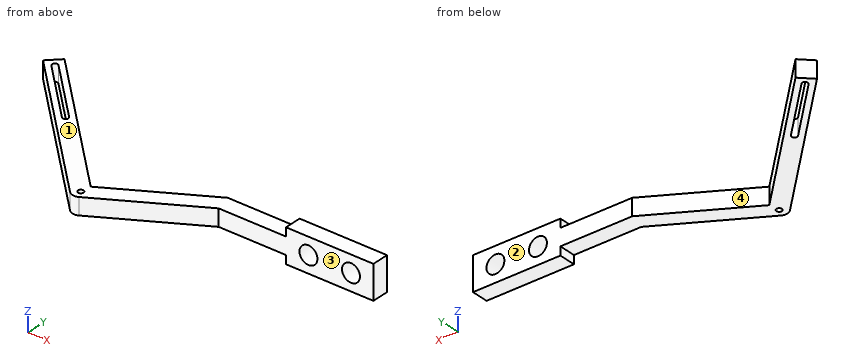
Autodesk Inventor part; units mm, degrees
ref_plane "YZ Plane" through (0, 0, 0) normal (1, 0, 0) x (0, 1, 0)
ref_plane "XZ Plane" through (0, 0, 0) normal (0, 1, 0) x (-1, 0, 0)
ref_plane "XY Plane" through (0, 0, 0) normal (0, 0, 1) x (1, 0, 0)
sketch "Sketch1" plane through (0, 0, 0) normal (0, 0, 1) x (1, 0, 0)
  line L0 (37.3205, 11.5) -> (16.9186, 11.5)
  line L1 (-26.163, 24.0416) -> (-1.0607, -1.0607)
  line L2 (17.7224, 8.5) -> (0.75, -1.299)
  line L3 (17.7224, 8.5) -> (37.3205, 8.5)
  line L4 (0.2468, 1.8745) -> (16.9186, 11.5)
  line L5 (0.2468, 1.8745) -> (-24.0416, 26.163)
  arc A0 (-23.6881, 24.3952) -> (-24.3952, 23.6881) centre (-24.0416, 24.0416) ccw
  arc A1 (-14.4957, 13.7886) -> (-13.7886, 14.4957) centre (-14.1421, 14.1421) ccw
  circle A2 centre (0, 0) radius 0.5
  line L6 (-25.1023, 25.1023) -> (-26.163, 24.0416)
  line L7 (-24.0416, 26.163) -> (-25.1023, 25.1023)
  line L8 (-24.3952, 23.6881) -> (-14.4957, 13.7886)
  line L9 (-13.7886, 14.4957) -> (-23.6881, 24.3952)
  line L10 (37.3205, 8.5) -> (45.3205, 8.5)
  line L11 (45.3205, 8.5) -> (45.3205, 11.5)
  line L12 (45.3205, 11.5) -> (37.3205, 11.5)
  arc A3 (-1.0607, -1.0607) -> (0.75, -1.299) centre (0, 0) ccw
extrude "Extrusion1" add sketch "Sketch1" along normal blind 3
sketch "Sketch5" plane through (0, 0, 3) normal (0, 0, 1) x (1, 0, 0)
  point P0 (0, 0)
sketch "Sketch8" plane through (45.3205, 8.5, 0) normal (1, 0, 0) x (0, 0, -1)
  line L0 (0, 0) -> (-3, 0)
  line L1 (-3, 0) -> (-4.5, 0)
  line L2 (-4.5, 0) -> (-4.5, 3)
  line L3 (-4.5, 3) -> (1.5, 3)
  line L4 (1.5, 3) -> (1.5, 0)
  line L5 (1.5, 0) -> (-3, 0)
  point P0 (0, -8.5)
  dimension "d38" = 1.5
  dimension "d39" = 3
  dimension "d40" = 6
  dimension "d41" = 3
extrude "Extrusion4" add sketch "Sketch8" against normal blind 15.588
sketch "Sketch9" plane through (16.9186, 11.5, 3) normal (0, 1, 0) x (1, 0, 0)
  line L0 (28.4019, 4.5) -> (28.4019, -1.5) construction
  point P0 (-16.9186, 3)
  point P1 (24.4019, 1.5)
  point P2 (16.8139, 1.5)
hole "Hole2" at (41.3205, 11.5, 1.5) at (33.7325, 11.5, 1.5) direction (0, -1, 0) diameter 3.2 end through all
properties part number "Ramię♥" material "Stainless Steel, Austenitic"
Part model, mm, in its own coordinate system. Face numbers are marked on the shaded views. A direction names the side the tool comes from. Round coordinates to 2 decimals unless told otherwise and drop trailing zeros. Write each loop counter-clockwise with the first axis right and the second up, starting at its lowest first coordinate (ties: lowest second). Pieces come first, ordered by that corner, then holes.
Item 1: Cut at D-D, the plane x = 28.5. Give the cut face in (y, z), plus the area to 3 significant figures.
Results:
outline: (8.5, 0) - (11.5, 0) - (11.5, 3) - (8.5, 3) - close
area: 9.00 mm2
Item 2: Drop flat-ended pins along their axis: pin 1 Ø1.2 at (y, z) = (9.5, -1) entering from -X; pin 2 Ø2 at (x, z) = (37.5, 0.5) entering from +Y; pin 3 Ø3 at (x, z) = (31, 2.5) entering from -Y. Give the stop position or say it passes through.
Results:
pin 1: stops at x = 29.73
pin 2: stops at y = 11.5
pin 3: stops at y = 8.5
Item 3: Probe L1, parallel to X at y = 10.25, z = 1.5; L2, parallel to X at y = 9.2, z = 1.5; L3, parallel to X at y = 8.25, z = 0.75. List the from-to ranges inside material, lowest first.
Results:
L1: x = -12.37 to -8.13, 14.75 to 32.13, 35.33 to 39.72, 42.92 to 45.32
L2: x = -11.32 to -7.08, 12.93 to 32.13, 35.33 to 39.72, 42.92 to 45.32
L3: x = -10.37 to -6.13, 11.29 to 17.29
Item 4: Which spindle directions (+Z, -Z, +X, -X, +Y, -Y) get a long thin tool onto all of the face, cutting with end or side? Do the marked faces 1, 2, 3 and 4. Say none if no direction does.
Results:
face 1: +Z, -X, +Y, -Y
face 2: +Z, -Z, +X, +Y
face 3: +Z, -Z, +X, -Y
face 4: +Z, -Z, +Y
Item 5: Cut at B-B, the plane y = 21.75. Give the cut face in (x, z).
Results:
outline: (-23.87, 0) - (-22.46, 0) - (-22.46, 3) - (-23.87, 3) - close; (-21.04, 0) - (-19.63, 0) - (-19.63, 3) - (-21.04, 3) - close
Item 6: Cut at A-A, the plane z = 1.5. Give the cut face in (x, y), plus the area to 3 significant figures.
Results:
outline: (-26.16, 24.04) - (-1.06, -1.06) arc R1.5 ccw to (0.75, -1.3) - (17.72, 8.5) - (32.13, 8.5) - (32.13, 11.5) - (16.92, 11.5) - (0.25, 1.87) - (-24.04, 26.16) - close; (35.33, 8.5) - (39.72, 8.5) - (39.72, 11.5) - (35.33, 11.5) - close; (42.92, 8.5) - (45.32, 8.5) - (45.32, 11.5) - (42.92, 11.5) - close; hole (-24.4, 23.69) - (-14.5, 13.79) arc R0.5 ccw to (-13.79, 14.5) - (-23.69, 24.4) arc R0.5 ccw to start; hole circle Ø1 at (0, 0)
area: 215 mm2
Item 7: Cut at C-C, the plane y = 10.75. Give the cut face in (x, z), plus the area to 3 significant figures.
Results:
outline: (-12.87, 0) - (-8.63, 0) - (-8.63, 3) - (-12.87, 3) - close; (15.62, 0) - (29.73, 0) - (29.73, -1.5) - (45.32, -1.5) - (45.32, 4.5) - (29.73, 4.5) - (29.73, 3) - (15.62, 3) - close; hole circle Ø3.2 at (33.73, 1.5); hole circle Ø3.2 at (41.32, 1.5)
area: 133 mm2
